The listing builds one solid part. Answer for the finished solid, in the listing's coordinates (mm). Face numbers are marked on the shaded views. A direction names the side the tool comes from. Round coordinates to 2 decimals unless told otherwise and drop trailing zeros. Loops run counter-clockwise (first coordinate to the right, second up) from the corner with the lowest first, then second, coordinate; pieces in that order, holes last. Notation, with made-up numbers: (-8.5, -23.5) -> (8.5, -23.5) arc R17 ccw to (8.5, 6.5) -> close; hole circle Ø4 at (-28, 82.25). An arc over 180 degrees is marked (long way). Write each question's results on one line, items separated by ' | '. Start each with the question number.
(1) The part is cut by section B-B (x = 0.25). Determine the outline of the cut face in (y, z), plus the area to 3 significant figures.
(2) The part is cut by section D-D (x = -6.25). Determine the outline of the cut face in (y, z).
(3) The part is cut by section C-C (y = -11). Determine the outline of the cut face in (x, z), plus the area to 3 significant figures.
(4) Flat-ended cylindrical pins translate along their axes: pin 1 (2.5 mm diameter, centred on x = -3.5, z = 1.5, fed in from -Y); pin 2 (4 mm diameter, centred on x = -0.6, y = -11.57, fed in from +Z); pin 3 (1.6 mm diameter, centred on y = -29.5, z = 1.5, fed in from -X); pin 4 (1.6 mm diameter, centred on y = -28.5, z = -19.5, fed in from +X). Find the tip coordinate at first contact, or state that the pin passes through.
(5) Determine the mould class of the marked faces 1, 2, 3 and 4 for opening direction X: released by +X, released by -X, zero draft, split by the parting line, or undercut.
(6) Straight lines are drawn through the part: probe 1 along Z at (x, y) = (-0.25, -37); probe 2 along Z at (x, y) = (-8.25, -2); probe 3 along Y at (x, z) = (-5, -11.25). For each, find the intervals that lie inside material, in ascending order.
(7) The part is cut by section A-A (y = -34). Determine the outline of the cut face in (x, z).
(8) For the marked faces 5 and 6, determine the directions among +Z, -Z, +X, -X, +Y, -Y from which every point of the face is accessible in a straight line to the end or side of a thin tool.
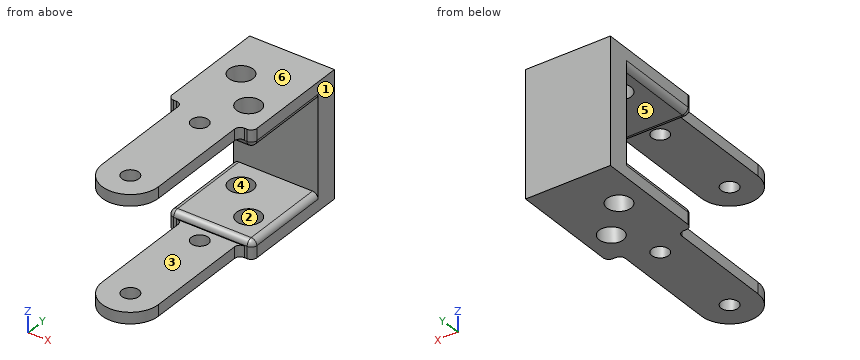
```python
from build123d import *

# Parameters (mm, degrees)
BOSS_EXTRUDE1_START   = 0.1
SKETCH1_R             = 1.5
BOSS_EXTRUDE1_DEPTH   = 2
SKETCH2_W             = 15
SKETCH2_H             = 3.1
SKETCH2_W_2           = 10
SKETCH2_H_2           = 2
BOSS_EXTRUDE2_DEPTH   = 16
SKETCH3_W             = 15
SKETCH3_H             = 22.2
BOSS_EXTRUDE3_DEPTH   = 4
BOSS_EXTRUDE4_START   = -20.1
SKETCH1_3_R           = 1.5
BOSS_EXTRUDE4_DEPTH   = 2
FILLET1_R             = 1
FILLET2_R             = 1
F_4_0MM_DOWEL_HOLE1_D = 4.3


with BuildPart() as part:
    # Sketch1 → Boss-Extrude1 (new body)
    with BuildSketch(Plane.XY.offset(BOSS_EXTRUDE1_START)):
        with BuildLine():
            Line((-8.650697236, -36.32930415), (-8.650697236, -16.72930415))
            Line((-8.650697236, -16.72930415), (1.349302764, -16.72930415))
            Line((1.349302764, -16.72930415), (1.349302764, -36.32930415))
            ThreePointArc((1.349302764, -36.32930415), (-3.650697236, -41.32930415), (-8.650697236, -36.32930415))
        make_face()
        with Locations((-3.650697236, -19.32930415)):
            Circle(SKETCH1_R, mode=Mode.SUBTRACT)
        with Locations((-3.650697236, -36.32930415)):
            Circle(SKETCH1_R, mode=Mode.SUBTRACT)
    extrude(amount=BOSS_EXTRUDE1_DEPTH)

    # Sketch2 → Boss-Extrude2 (add)
    with BuildSketch(Plane(origin=(0, -16.72930415, 0), x_dir=(1, 0, 0), z_dir=(0, 1, 0))):
        with Locations((-3.650697236, 18.55)):
            Rectangle(SKETCH2_W, SKETCH2_H)
        Polygon((3.849302764, 1), (-11.150697236, 1), (-11.150697236, -2.1), (-8.650697236, -2.1), (-8.650697236, -0.1), (1.349302764, -0.1), (1.349302764, -2.1), (3.849302764, -2.1), align=None)
        with Locations((-3.650697236, -1.1)):
            Rectangle(SKETCH2_W_2, SKETCH2_H_2)
    extrude(amount=BOSS_EXTRUDE2_DEPTH)

    # Sketch3 → Boss-Extrude3 (add)
    with BuildSketch(Plane(origin=(0, -0.72930415, 0), x_dir=(1, 0, 0), z_dir=(0, 1, 0))):
        with Locations((-3.650697236, 9)):
            Rectangle(SKETCH3_W, SKETCH3_H)
    extrude(amount=BOSS_EXTRUDE3_DEPTH)

    # Sketch1<3> → Boss-Extrude4 (add)
    with BuildSketch(Plane.XY.offset(BOSS_EXTRUDE4_START)):
        with BuildLine():
            Line((-8.650697236, -36.32930415), (-8.650697236, -16.72930415))
            Line((-8.650697236, -16.72930415), (1.349302764, -16.72930415))
            Line((1.349302764, -16.72930415), (1.349302764, -36.32930415))
            ThreePointArc((1.349302764, -36.32930415), (-3.650697236, -41.32930415), (-8.650697236, -36.32930415))
        make_face()
        with Locations((-3.650697236, -19.32930415)):
            Circle(SKETCH1_3_R, mode=Mode.SUBTRACT)
        with Locations((-3.650697236, -36.32930415)):
            Circle(SKETCH1_3_R, mode=Mode.SUBTRACT)
    extrude(amount=BOSS_EXTRUDE4_DEPTH)

    # Fillet1
    fillet1_edges = [part.edges().sort_by_distance(p)[0] for p in [
        (3.849302764, -16.72930415, 0.55),
        (-11.150697236, -16.72930415, 0.55),
        (3.849302764, -16.72930415, -18.55),
        (-11.150697236, -16.72930415, -18.55),
        (-8.650697236, -16.72930415, -19.1),
        (1.349302764, -16.72930415, -19.1),
        (-8.650697236, -16.72930415, 1.1),
        (1.349302764, -16.72930415, 1.1),
    ]]
    fillet(fillet1_edges, radius=FILLET1_R)

    # Fillet2
    fillet2_edges = [part.edges().sort_by_distance(p)[0] for p in [
        (-11.150697236, -8.22930415, -1),
        (3.849302764, -8.22930415, -1),
        (-11.150697236, -8.22930415, -17),
        (3.849302764, -8.22930415, -17),
        (-3.650697236, -16.72930415, -17),
        (-10.857804017, -16.436410931, -17),
        (3.556409546, -16.436410931, -17),
        (-3.650697236, -16.72930415, -1),
        (3.556409546, -16.436410931, -1),
        (-10.857804017, -16.436410931, -1),
    ]]
    fillet(fillet2_edges, radius=FILLET2_R)

    # Ø4.0mm Dowel Hole1 (through all)
    with Locations(Plane(origin=(-6.364117909, -5.47483866, -20.1), x_dir=(-1, 0, 0), z_dir=(0, 0, -1))):
        with Locations((0, 0), (-5.759484696, -6.093076476)):
            Hole(F_4_0MM_DOWEL_HOLE1_D / 2)


solid = part.part
```
Checked values:
1) outline: (-39.46, -20.1) -> (-13.54, -20.1) -> (-13.54, -17) -> (-15.73, -17) arc R1 ccw to (-16.73, -18) -> (-16.73, -18.1) -> (-39.46, -18.1) -> close; (-39.46, 0.1) -> (-16.73, 0.1) -> (-16.73, 0) arc R1 ccw to (-15.73, -1) -> (-13.54, -1) -> (-13.54, 2.1) -> (-39.46, 2.1) -> close; (-9.6, -20.1) -> (3.27, -20.1) -> (3.27, 2.1) -> (-9.6, 2.1) -> (-9.6, -1) -> (-0.73, -1) -> (-0.73, -17) -> (-9.6, -17) -> close | area: 254 mm2
2) outline: (-40.6, -20.1) -> (-7.62, -20.1) -> (-7.62, -17) -> (-15.73, -17) arc R1 ccw to (-16.73, -18) -> (-16.73, -18.1) -> (-40.6, -18.1) -> close; (-40.6, 0.1) -> (-16.73, 0.1) -> (-16.73, 0) arc R1 ccw to (-15.73, -1) -> (-7.62, -1) -> (-7.62, 2.1) -> (-40.6, 2.1) -> close; (-3.33, -20.1) -> (3.27, -20.1) -> (3.27, 2.1) -> (-3.33, 2.1) -> (-3.33, -1) -> (-0.73, -1) -> (-0.73, -17) -> (-3.33, -17) -> close
3) outline: (-11.15, -20.1) -> (-2.68, -20.1) -> (-2.68, -17) -> (-10.15, -17) arc R1 ccw to (-11.15, -18) -> close; (-11.15, 0) arc R1 ccw to (-10.15, -1) -> (-2.68, -1) -> (-2.68, 2.1) -> (-11.15, 2.1) -> close; (1.47, -20.1) -> (3.85, -20.1) -> (3.85, -18) arc R1 ccw to (2.85, -17) -> (1.47, -17) -> close; (1.47, -1) -> (2.85, -1) arc R1 ccw to (3.85, 0) -> (3.85, 2.1) -> (1.47, 2.1) -> close | area: 66.4 mm2
4) pin 1: stops at y = -41.33 | pin 2: passes through | pin 3: stops at x = -8.65 | pin 4: stops at x = 1.35
5) face 1: released by +X | face 2: undercut | face 3: zero draft | face 4: undercut
6) probe 1: z = -20.1 to -18.1, 0.1 to 2.1 | probe 2: z = -20.1 to -17, -1 to 2.1 | probe 3: y = -0.73 to 3.27
7) outline: (-8.65, -20.1) -> (1.35, -20.1) -> (1.35, -18.1) -> (-8.65, -18.1) -> close; (-8.65, 0.1) -> (1.35, 0.1) -> (1.35, 2.1) -> (-8.65, 2.1) -> close
8) face 5: +X, -X, -Y | face 6: +Z, +X, -X, +Y, -Y
